For this review, take the finished solid that the model builds, in its own axes (mm). A direction names the side the tool comes from. Give positions to 0.01 mm unless a question says otherwise; leave off trailing zeros. Order: outer loops, then holes, each group sorted by start corner. A loop starts at its lowest first (then second) coordinate and runs counter-clockwise, first axis right, second up. Notation, with made-up numbers: M -31,23.25 L 9,23.25 A28 ccw 9,52.25 Z; hole C -10,-9.75 d9. An arc over 180 degrees is marked long. Use CSV: the item, a comma, the result in double quotes. Start each with the question number.
(1) Wall thickness on L1, parallel to X at y = -1, z = -19.5: over which ranges is the line inside the solid? List them lowest first. Write a range as from..to.
(2) Consider section D-D (z = 12.5). Write out the cut boundary in (x, y), and give its area (3 significant figures).
(3) Clearance check with flat-ended pins moving along their axes: P1, Ø3, axis at x = 5.5, z = 2, coming from the +Y side; P2, Ø14, axis at y = -8.5, z = 18.5, coming from the +X side; P3, Ø3.5, axis at x = 26, y = 1.5, coming from the -Z side. State where each tip first meets the part, or that it passes through.
(4) Consider section A-A (z = 0). Write out the cut boundary in (x, y), and give its area (3 significant figures).
(5) Tool access review of faces 1 (the face through (1.479, -14.79, -15.465)), 2 (the face through (25.73, 1.48, 25.18)): name each direction out of +Z, -Z, +X, -X, +Y, -Y from which nothing blocks a thin tool from reaching the whole face with its end or side.
(6) Consider section B-B (x = 24). Write out the cut boundary in (y, z), and give its area (3 significant figures).
(7) Draft analysis for pull direction Z (two halves, no side actions). For faces 3 (the face through (4, -30, 0)), 4 (the face through (10, -29, 0)), 5 (the face through (1.48, -13.69, -12.86)), state which applies: pulls with the +Z half, pulls with the -Z half, needs draft (parallel to the pull), parting line crosses it, or undercut.
(8) Consider section C-C (x = 9). Write out the cut boundary in (y, z), and give its area (3 significant figures).
```python
from build123d import *

# Parameters (mm, degrees)
BOSS_EXTRUDE2_DEPTH = 3
BOSS_EXTRUDE3_DEPTH = 3
BOSS_EXTRUDE4_DEPTH = 3


with BuildPart() as part:
    # Sketch1 → Boss-Extrude2 (new body)
    with BuildSketch(Plane(origin=(0, 0, 0), x_dir=(1, 0, 0), z_dir=(0, 1, 0))):
        with BuildLine():
            Line((0, -17.78), (0, -38.5))
            ThreePointArc((0, -38.5), (38.5, 0), (0, 38.5))
            Line((0, 38.5), (0, 17.78))
            ThreePointArc((0, 17.78), (17.78, 0), (0, -17.78))
        make_face()
        with BuildLine():
            Line((3, 35.874782229), (3, 19.652338283))
            ThreePointArc((3, 19.652338283), (14.580910151, 13.513380746), (19.82332969, 1.5))
            Line((19.82332969, 1.5), (35.968736425, 1.5))
            ThreePointArc((35.968736425, 1.5), (25.981666959, 24.918928188), (3, 35.874782229))
        make_face(mode=Mode.SUBTRACT)
        with BuildLine():
            Line((3, -19.652338283), (3, -35.874782229))
            ThreePointArc((3, -35.874782229), (25.981666959, -24.918928188), (35.968736425, -1.5))
            Line((35.968736425, -1.5), (19.82332969, -1.5))
            ThreePointArc((19.82332969, -1.5), (14.580910151, -13.513380746), (3, -19.652338283))
        make_face(mode=Mode.SUBTRACT)
    extrude(amount=BOSS_EXTRUDE2_DEPTH)



with BuildPart() as body_2:
    # Sketch4 → Boss-Extrude3 (new body)
    with BuildSketch(Plane(origin=(0, -30, 0), x_dir=(-1, 0, 0), z_dir=(0, -1, 0))):
        with BuildLine():
            Line((0, 10), (0, -10))
            ThreePointArc((0, -10), (-10, 0), (0, 10))
        make_face()
    extrude(amount=-BOSS_EXTRUDE3_DEPTH)


with BuildPart() as part_1:
    add(part.part)

    add(body_2.part)  # Boss-Extrude4 merges body 2
    # Sketch6 → Boss-Extrude4 (add)
    with BuildSketch(Plane(origin=(0, 0, 0), x_dir=(0, 0, -1), z_dir=(1, 0, 0))):
        Polygon((20.78, 0), (10, -30), (8.078, -30), (8.078, -27), (17.78, 0), align=None)
        Polygon((-20.974429694, 0), (-10, -30), (-7.903013275, -30), (-7.903013275, -27), (-17.78, 0), align=None)
    extrude(amount=BOSS_EXTRUDE4_DEPTH)


solid = part_1.part
```
Check result:
1,L1,"x = 0..3"
2,outline,"M 0,-23.17 L 3,-23.17 L 3,-14.43 L 0,-14.43 Z; M 12.64,0 L 15.46,0 L 15.46,3 L 12.64,3 Z; M 33.76,0 L 36.41,0 L 36.41,3 L 33.76,3 Z"
2,area,"42.6 mm^2"
3,P1,"stops at y = -27"
3,P2,"stops at x = 3"
3,P3,"stops at z = -29.9"
4,outline,"M 0,-30 L 10,-30 L 10,-27 L 0,-27 Z; M 17.78,0 L 38.5,0 L 38.5,3 L 17.78,3 Z"
4,area,"92.2 mm^2"
5,face 1,"-Z, +X, -X, -Y"
5,face 2,"+Y, -Y"
6,outline,"M 0,-30.1 L 3,-30.1 L 3,-26.83 L 0,-26.83 Z; M 0,-1.5 L 3,-1.5 L 3,1.5 L 0,1.5 Z; M 0,26.83 L 3,26.83 L 3,30.1 L 0,30.1 Z"
6,area,"28.6 mm^2"
7,face 3,"needs draft"
7,face 4,"parting line crosses it"
7,face 5,"undercut"
8,outline,"M -30,-4.36 L -27,-4.36 L -27,4.36 L -30,4.36 Z; M 0,-37.43 L 3,-37.43 L 3,-34.86 L 0,-34.86 Z; M 0,-17.73 L 3,-17.73 L 3,-15.33 L 0,-15.33 Z; M 0,15.33 L 3,15.33 L 3,17.73 L 0,17.73 Z; M 0,34.86 L 3,34.86 L 3,37.43 L 0,37.43 Z"
8,area,"56.0 mm^2"
